from build123d import *

# Parameters (mm, degrees)
BOSS_EXTRUDE1_DEPTH   = 3
BOSS_EXTRUDE1_2_DEPTH = 3
BOSS_EXTRUDE1_3_DEPTH = 3
BOSS_EXTRUDE1_4_DEPTH = 3
BOSS_EXTRUDE2_START   = -3
SKETCH2_R             = 11.25
BOSS_EXTRUDE2_DEPTH   = 3
CUT_EXTRUDE1_REACH    = 76.288
SKETCH3_R             = 1.5
FILLET1_R             = 2
SKETCH4_R             = 14.25
SKETCH4_R_2           = 11.25
BOSS_EXTRUDE3_DEPTH   = 5
FILLET3_R             = 2
FILLET2_R             = 3
CUT_EXTRUDE2_REACH    = 76.396
SKETCH6_R             = 1.5
FILLET4_R             = 2
CUT_EXTRUDE3_REACH    = 76.396
SKETCH7_R             = 1.5
FILLET5_R             = 2
CUT_EXTRUDE4_REACH    = 75.948
SKETCH8_R             = 1.5
FILLET6_R             = 2
FILLET7_R             = 3
FILLET8_R             = 20


with BuildPart() as part:
    # Sketch1 → Boss-Extrude1 (new body)
    with BuildSketch(Plane(origin=(0, 0, 0), x_dir=(1, 0, 0), z_dir=(0, 1, 0))):
        with BuildLine():
            Line((-34.371558273, -36.312476945), (-38.95676142, -42.247619075))
            Line((-38.95676142, -42.247619075), (-31.04323858, -48.361223271))
            Line((-31.04323858, -48.361223271), (-26.458035433, -42.426081141))
            ThreePointArc((-26.458035433, -42.426081141), (-30.568020981, -39.567614198), (-34.371558273, -36.312476945))
        make_face()
    extrude(amount=BOSS_EXTRUDE1_DEPTH)



with BuildPart() as body_2:
    # Sketch1 → Boss-Extrude1 2 (new body)
    with BuildSketch(Plane(origin=(0, 0, 0), x_dir=(1, 0, 0), z_dir=(0, 1, 0))):
        with BuildLine():
            Line((14.261748373, -47.922881104), (17.109130658, -54.861354576))
            Line((17.109130658, -54.861354576), (26.360428621, -51.064844862))
            Line((26.360428621, -51.064844862), (23.513046335, -44.12637139))
            ThreePointArc((23.513046335, -44.12637139), (18.982548572, -46.256489812), (14.261748373, -47.922881104))
        make_face()
    extrude(amount=BOSS_EXTRUDE1_2_DEPTH)


with BuildPart() as body_3:
    # Sketch1 → Boss-Extrude1 3 (new body)
    with BuildSketch(Plane(origin=(0, 0, 0), x_dir=(1, 0, 0), z_dir=(0, 1, 0))):
        with BuildLine():
            Line((34.371558273, 36.312476945), (38.95676142, 42.247619075))
            Line((38.95676142, 42.247619075), (31.04323858, 48.361223271))
            Line((31.04323858, 48.361223271), (26.458035433, 42.426081141))
            ThreePointArc((26.458035433, 42.426081141), (30.568020981, 39.567614198), (34.371558273, 36.312476945))
        make_face()
    extrude(amount=BOSS_EXTRUDE1_3_DEPTH)


with BuildPart() as body_4:
    # Sketch1 → Boss-Extrude1 4 (new body)
    with BuildSketch(Plane(origin=(0, 0, 0), x_dir=(1, 0, 0), z_dir=(0, 1, 0))):
        with BuildLine():
            Line((-14.261748373, 47.922881104), (-17.109130658, 54.861354576))
            Line((-17.109130658, 54.861354576), (-26.360428621, 51.064844862))
            Line((-26.360428621, 51.064844862), (-23.513046335, 44.12637139))
            ThreePointArc((-23.513046335, 44.12637139), (-18.982548572, 46.256489812), (-14.261748373, 47.922881104))
        make_face()
    extrude(amount=BOSS_EXTRUDE1_4_DEPTH)


with BuildPart() as part_1:
    add(part.part)

    add(body_2.part)  # Boss-Extrude2 merges body 2

    add(body_3.part)  # Boss-Extrude2 merges body 3

    add(body_4.part)  # Boss-Extrude2 merges body 4
    # Sketch2 → Boss-Extrude2 (add)
    with BuildSketch(Plane(origin=(0, 3, 0), x_dir=(1, 0, 0), z_dir=(0, 1, 0)).offset(BOSS_EXTRUDE2_START)):
        with BuildLine():
            Line((-26.458035433, -42.426081141), (14.261748373, -47.922881104))
            ThreePointArc((14.261748373, -47.922881104), (18.982548572, -46.256489812), (23.513046335, -44.12637139))
            ThreePointArc((23.513046335, -44.12637139), (8.334035055, -1.125018831), (34.371558273, 36.312476945))
            ThreePointArc((34.371558273, 36.312476945), (30.568020981, 39.567614198), (26.458035433, 42.426081141))
            Line((26.458035433, 42.426081141), (-14.261748373, 47.922881104))
            ThreePointArc((-14.261748373, 47.922881104), (-18.982548572, 46.256489812), (-23.513046335, 44.12637139))
            ThreePointArc((-23.513046335, 44.12637139), (-49.550569553, 6.688875614), (-34.371558273, -36.312476945))
            ThreePointArc((-34.371558273, -36.312476945), (-30.568020981, -39.567614198), (-26.458035433, -42.426081141))
        make_face()
        with Locations(Location((-30, 0, 0), (0, 0, 270))):
            Circle(SKETCH2_R, mode=Mode.SUBTRACT)
    extrude(amount=BOSS_EXTRUDE2_DEPTH)

    # Sketch3 → Cut-Extrude1 (cut, up to next)
    with BuildSketch(Plane(origin=(0, 3, 0), x_dir=(1, 0, 0), z_dir=(0, 1, 0)), mode=Mode.PRIVATE) as cut_extrude1_sk1:
        with Locations(Location((-35.297139556, -41.599801343, 0), (0, 0, 270))):
            Circle(SKETCH3_R)
    cut_extrude1_tool1 = extrude(cut_extrude1_sk1.sketch, amount=-CUT_EXTRUDE1_REACH, mode=Mode.PRIVATE) & part_1.part
    # Sketch3 → Cut-Extrude1 (cut, up to next)
    with BuildSketch(Plane(origin=(0, 3, 0), x_dir=(1, 0, 0), z_dir=(0, 1, 0)), mode=Mode.PRIVATE) as cut_extrude1_sk2:
        with Locations(Location((-31.340378136, -44.656603441, 0), (0, 0, 270))):
            Circle(SKETCH3_R)
    cut_extrude1_tool2 = extrude(cut_extrude1_sk2.sketch, amount=-CUT_EXTRUDE1_REACH, mode=Mode.PRIVATE) & part_1.part
    add(cut_extrude1_tool1.solids().sort_by_distance((-35.29714, 3, 41.599801))[0], mode=Mode.SUBTRACT)
    add(cut_extrude1_tool2.solids().sort_by_distance((-31.340378, 3, 44.656603))[0], mode=Mode.SUBTRACT)

    # Fillet1
    fillet1_edges = [part_1.edges().sort_by_distance(p)[0] for p in [
        (-31.04323858, 1.5, 48.361223271),
        (-38.95676142, 1.5, 42.247619075),
    ]]
    fillet(fillet1_edges, radius=FILLET1_R)

    # Sketch4 → Boss-Extrude3 (add)
    with BuildSketch(Plane(origin=(0, 3, 0), x_dir=(1, 0, 0), z_dir=(0, 1, 0))):
        with Locations(Location((-30, 0, 0), (0, 0, 270))):
            Circle(SKETCH4_R)
        with Locations(Location((-30, 0, 0), (0, 0, 270))):
            Circle(SKETCH4_R_2, mode=Mode.SUBTRACT)
    extrude(amount=BOSS_EXTRUDE3_DEPTH)

    # Fillet3
    fillet3_edges = [part_1.edges().sort_by_distance(p)[0] for p in [
        (-30, 8, -11.25),
    ]]
    fillet(fillet3_edges, radius=FILLET3_R)

    # Fillet2
    fillet2_edges = [part_1.edges().sort_by_distance(p)[0] for p in [
        (-30, 3, -14.25),
    ]]
    fillet(fillet2_edges, radius=FILLET2_R)

    # Sketch6 → Cut-Extrude2 (cut, up to next)
    with BuildSketch(Plane(origin=(0, 3, 0), x_dir=(1, 0, 0), z_dir=(0, 1, 0)), mode=Mode.PRIVATE) as cut_extrude2_sk1:
        with Locations(Location((18.377914978, -51.368120208, 0), (0, 0, 270))):
            Circle(SKETCH6_R)
    cut_extrude2_tool1 = extrude(cut_extrude2_sk1.sketch, amount=-CUT_EXTRUDE2_REACH, mode=Mode.PRIVATE) & part_1.part
    # Sketch6 → Cut-Extrude2 (cut, up to next)
    with BuildSketch(Plane(origin=(0, 3, 0), x_dir=(1, 0, 0), z_dir=(0, 1, 0)), mode=Mode.PRIVATE) as cut_extrude2_sk2:
        with Locations(Location((23.003563959, -49.469865351, 0), (0, 0, 270))):
            Circle(SKETCH6_R)
    cut_extrude2_tool2 = extrude(cut_extrude2_sk2.sketch, amount=-CUT_EXTRUDE2_REACH, mode=Mode.PRIVATE) & part_1.part
    add(cut_extrude2_tool1.solids().sort_by_distance((18.377915, 3, 51.36812))[0], mode=Mode.SUBTRACT)
    add(cut_extrude2_tool2.solids().sort_by_distance((23.003564, 3, 49.469865))[0], mode=Mode.SUBTRACT)

    # Fillet4
    fillet4_edges = [part_1.edges().sort_by_distance(p)[0] for p in [
        (17.109130658, 1.5, 54.861354576),
        (26.360428621, 1.5, 51.064844862),
    ]]
    fillet(fillet4_edges, radius=FILLET4_R)

    # Sketch7 → Cut-Extrude3 (cut, up to next)
    with BuildSketch(Plane(origin=(0, 3, 0), x_dir=(1, 0, 0), z_dir=(0, 1, 0)), mode=Mode.PRIVATE) as cut_extrude3_sk1:
        with Locations(Location((-18.377914978, 51.368120208, 0), (0, 0, 270))):
            Circle(SKETCH7_R)
    cut_extrude3_tool1 = extrude(cut_extrude3_sk1.sketch, amount=-CUT_EXTRUDE3_REACH, mode=Mode.PRIVATE) & part_1.part
    # Sketch7 → Cut-Extrude3 (cut, up to next)
    with BuildSketch(Plane(origin=(0, 3, 0), x_dir=(1, 0, 0), z_dir=(0, 1, 0)), mode=Mode.PRIVATE) as cut_extrude3_sk2:
        with Locations(Location((-23.003563959, 49.469865351, 0), (0, 0, 270))):
            Circle(SKETCH7_R)
    cut_extrude3_tool2 = extrude(cut_extrude3_sk2.sketch, amount=-CUT_EXTRUDE3_REACH, mode=Mode.PRIVATE) & part_1.part
    add(cut_extrude3_tool1.solids().sort_by_distance((-18.377915, 3, -51.36812))[0], mode=Mode.SUBTRACT)
    add(cut_extrude3_tool2.solids().sort_by_distance((-23.003564, 3, -49.469865))[0], mode=Mode.SUBTRACT)

    # Fillet5
    fillet5_edges = [part_1.edges().sort_by_distance(p)[0] for p in [
        (-17.109130658, 1.5, -54.861354576),
        (-26.360428621, 1.5, -51.064844862),
    ]]
    fillet(fillet5_edges, radius=FILLET5_R)

    # Sketch8 → Cut-Extrude4 (cut, up to next)
    with BuildSketch(Plane(origin=(0, 3, 0), x_dir=(1, 0, 0), z_dir=(0, 1, 0)), mode=Mode.PRIVATE) as cut_extrude4_sk1:
        with Locations(Location((35.297139556, 41.599801343, 0), (0, 0, 270))):
            Circle(SKETCH8_R)
    cut_extrude4_tool1 = extrude(cut_extrude4_sk1.sketch, amount=-CUT_EXTRUDE4_REACH, mode=Mode.PRIVATE) & part_1.part
    # Sketch8 → Cut-Extrude4 (cut, up to next)
    with BuildSketch(Plane(origin=(0, 3, 0), x_dir=(1, 0, 0), z_dir=(0, 1, 0)), mode=Mode.PRIVATE) as cut_extrude4_sk2:
        with Locations(Location((31.340378136, 44.656603441, 0), (0, 0, 270))):
            Circle(SKETCH8_R)
    cut_extrude4_tool2 = extrude(cut_extrude4_sk2.sketch, amount=-CUT_EXTRUDE4_REACH, mode=Mode.PRIVATE) & part_1.part
    add(cut_extrude4_tool1.solids().sort_by_distance((35.29714, 3, -41.599801))[0], mode=Mode.SUBTRACT)
    add(cut_extrude4_tool2.solids().sort_by_distance((31.340378, 3, -44.656603))[0], mode=Mode.SUBTRACT)

    # Fillet6
    fillet6_edges = [part_1.edges().sort_by_distance(p)[0] for p in [
        (38.95676142, 1.5, -42.247619075),
        (31.04323858, 1.5, -48.361223271),
    ]]
    fillet(fillet6_edges, radius=FILLET6_R)

    # Fillet7
    fillet7_edges = [part_1.edges().sort_by_distance(p)[0] for p in [
        (14.261748373, 1.5, 47.922881104),
        (26.458035433, 1.5, -42.426081141),
        (-14.261748373, 1.5, -47.922881104),
        (-23.513046335, 1.5, -44.12637139),
        (-26.458035433, 1.5, 42.426081141),
        (-34.371558273, 1.5, 36.312476945),
    ]]
    fillet(fillet7_edges, radius=FILLET7_R)

    # Fillet8
    fillet8_edges = [part_1.edges().sort_by_distance(p)[0] for p in [
        (23.513046335, 1.5, 44.12637139),
        (34.371558273, 1.5, -36.312476945),
    ]]
    fillet(fillet8_edges, radius=FILLET8_R)


solid = part_1.part
Read the model definition and answer for the solid it produces. Units are mm, in the model's axes. A direction names the side the tool comes from. Coordinates: 2 decimals unless noted, no trailing zeros. Write each loop counter-clockwise with the first axis right and the second up, starting at its lowest first coordinate (ties: lowest second). Pieces come first, ordered by that corner, then holes. Notation, with made-up numbers: (-17.75, 14.5) -> (41.25, 14.5) arc R23 ccw to (41.25, 49.5) -> close; hole circle Ø7 at (70, -27). An arc over 180 degrees is marked (long way). Return JSON: item names as keys, results as strings.
(1) Consider line 1 along Z through (x, y) = (-37, 2.75); line 2 along Y through (x, z) = (-34.5, -28); line 3 along Z through (x, y) = (-25, 6.75). Determine where each line is inside the solid, lowest interval first. Write a range as from..to.
Answers below:
{"line 1": "-33.63..-8.81, 8.81..33.63, 39.71..43.76", "line 2": "0..3", "line 3": "-13.34..-10.24, 10.24..13.34"}
(2) The part is cut by section C-C on x = 1. Give the vertices of the cut face in (y, z), then the cut area to 3 significant figures.
Answers below:
{"outline": "(0, -45.86) -> (3, -45.86) -> (3, 46.13) -> (0, 46.13) -> close", "area": "276 mm^2"}
(3) Each of these flat-tipped pins is pushed along its axis until it touches: P1, Ø1.5, axis at y = 3, z = -18, coming from the +X side; P2, Ø2.5, axis at x = 18.38, z = 51.37, coming from the -Y side; P3, Ø1, axis at x = -24.5, y = 6, coming from the -Z side; P4, Ø4, axis at x = 31.34, z = -44.66, coming from the +Y side. Where does it stop, or does it pass through?
Answers below:
{"P1": "x = 15.52", "P2": "through", "P3": "z = -13.34", "P4": "y = 3"}
(4) The part is cut by section D-D on z = -22. Give the vertices of the cut face in (x, y), then the cut area to 3 significant figures.
Answers below:
{"outline": "(-44.9, 0) -> (17.75, 0) -> (17.75, 3) -> (-44.9, 3) -> close", "area": "188 mm^2"}
(5) The part is cut by section B-B on y = 1.5. State how many separate pieces and enclosed holes the cut face has, then the cut area to 3 significant figures.
Answers below:
{"separate pieces": "1", "enclosed holes": "9", "area": "5,080 mm^2"}
(6) The part is cut by section A-A on z = 0. Give the vertices of the cut face in (x, y).
Answers below:
{"outline": "(-50, 0) -> (-41.25, 0) -> (-41.25, 6) arc R2 ccw to (-43.25, 8) -> (-44.25, 8) -> (-44.25, 6) arc R3 cw to (-47.25, 3) -> (-50, 3) -> close; (-18.75, 0) -> (8.5, 0) -> (8.5, 3) -> (-12.75, 3) arc R3 cw to (-15.75, 6) -> (-15.75, 8) -> (-16.75, 8) arc R2 ccw to (-18.75, 6) -> close"}
(7) For a pull along Z with two mould halves and no side action, classify faces 1 (the flat face through (-6.36, 1.48, 45.14)), 2 (the cylindrical face through (-13.961, 1.521, -48.277)), 3 (the cylindrical face through (-30.1, 1.5, 45.5)) as pulls with the +Z half, pulls with the -Z half, needs draft (parallel to the pull), parting line crosses it, or undercut.
Answers below:
{"face 1": "pulls with the +Z half", "face 2": "pulls with the -Z half", "face 3": "undercut"}
(8) Which of the six approach directions +Z, -Z, +X, -X, +Y, -Y give full straight-line access (tool end or side, diameter ignored) to faces 4 (the cylindrical face through (23.3, 1.5, 44.5)), 5 (the cylindrical face through (-40.982, 2.958, -2.439)), 6 (the flat face through (-36.85, 1.48, 39.52)), 7 (the flat face through (6.36, 1.48, -45.14)), 8 (the flat face through (-28.685, 1.479, 45.309))?
Answers below:
{"face 4": "+X, +Y, -Y", "face 5": "+Y, -Y", "face 6": "-X, +Y, -Y", "face 7": "-Z, +Y, -Y", "face 8": "+Z, +Y, -Y"}
